Design review of the part built by this model. Coordinates are the model's own, in mm. A direction names the side the tool comes from. Give positions to 0.01 mm unless a question says otherwise; leave off trailing zeros. Write each loop counter-clockwise with the first axis right and the second up, starting at its lowest first coordinate (ties: lowest second). Pieces come first, ordered by that corner, then holes. Notation, with made-up numbers: M 30,65 L 84,65 A12 cw 84,72 Z; hole C 0.25,81.5 d6. An arc over 180 degrees is marked long. Write each question's results on one line, items separated by ' | '. Start each with the question number.
Autodesk Inventor part; units mm, degrees
ref_plane "YZ Plane" through (0, 0, 0) normal (1, 0, 0) x (0, 1, 0)
ref_plane "XZ Plane" through (0, 0, 0) normal (0, 1, 0) x (-1, 0, 0)
ref_plane "XY Plane" through (0, 0, 0) normal (0, 0, 1) x (1, 0, 0)
sketch "Sketch1" plane through (0, 0, 0) normal (0, 0, 1) x (1, 0, 0)
  line L0 (0, 0) -> (-6.8, 0)
  line L1 (-6.8, 0) -> (-6.8, 2.775)
  line L2 (-6.8, 2.775) -> (-5.2, 2.775)
  line L3 (-5.2, 2.775) -> (-5.2, 1.5)
  line L4 (-5.2, 1.5) -> (6.8, 1.5)
  line L5 (6.8, 1.5) -> (6.8, 0)
  line L6 (6.8, 0) -> (0, 0)
  dimension "d0" = 12
  dimension "d1" = 2.775
  dimension "d2" = 1.6
  dimension "d3" = 1.5
revolve "Revolution1" add sketch "Sketch1" angle 360 about axis through (0, 0, 0) along (-1, 0, 0)
sketch "Sketch2" plane through (-6.8, 0, 0) normal (-1, 0, 0) x (0, 0, 1)
  line L0 (-1.1547, 0) -> (-0.5774, 1)
  line L1 (-0.5774, 1) -> (0.5774, 1)
  line L2 (0.5774, 1) -> (1.1547, 0)
  line L3 (1.1547, 0) -> (0.5774, -1)
  line L4 (0.5774, -1) -> (-0.5774, -1)
  line L5 (-0.5774, -1) -> (-1.1547, 0)
  point P0 (0, 0)
  point P1 (0, 0)
  dimension "d5" = 2
extrude "Extrusion1" cut sketch "Sketch2" against normal blind 1.5
properties part number "M3x12"
Q1. The part is to be moulded in two halves that separate along Y. For faces 1 (the flat face through (-6.06, 0.51, 0.86)), 2 (the cylindrical face through (0.88, -1.5, 0.07)), 3 (the flat face through (6.8, 0, 0)), say which applies: pulls with the +Y half, pulls with the -Y half, needs draft (parallel to the pull), parting line crosses it, or undercut.
Q2. We need section D-D on z = 2.05. Write out the cut boundary in (x, y).
Q3. We need section C-C on x = 4.75. Write out the cut boundary in (y, z), and give its area (3 significant figures).
Q4. We need section B-B on y = 0.85. Write out the cut boundary in (x, z).
Q5. Wall thickness on line 1 along X through (y, z) = (2.45, 0.55); line 2 along X through (y, z) = (0.5, 0.65); line 3 along Z through (x, y) = (-5.75, -0.6): over which ranges is each line inside the solid? List them lowest first. Write a range as from..to.
Q6. We need section A-A on z = 0. Write out the cut boundary in (x, y) (3 decimals).
Q7. For pin 1 Ø0.6 at (y, z) = (0, 0.5) entering from -X; pin 2 Ø2 at (x, z) = (0, -1) entering from +Y; pin 3 Ø2 at (y, z) = (1, 1.5) entering from +X; pin 4 Ø2 at (x, y) = (5, -0.5) entering from +Z, all flat-tipped, find the tip position at first contact; note any pin that passes through.
Q8. For faces 4 (the flat face through (-6, 1, 0)), 5 (the cylindrical face through (-5.99, 1.49, 2.34)), 6 (the flat face through (-5.2, 1.2, 1.2)), list the 3-axis set-ups (+Z, -Z, +X, -X, +Y, -Y) from which the entire face can be reached by the end or side of a thin tool; tool diameter is ignored.
Answer sheet:
1) face 1: undercut | face 2: parting line crosses it | face 3: needs draft
2) outline: M -6.8,-1.87 L -5.2,-1.87 L -5.2,1.87 L -6.8,1.87 Z
3) outline: C 0,0 d3 | area: 7.07 mm^2
4) outline: M -6.8,-2.64 L -5.2,-2.64 L -5.2,-1.24 L 6.8,-1.24 L 6.8,1.24 L -5.2,1.24 L -5.2,2.64 L -6.8,2.64 L -6.8,0.66 L -5.3,0.66 L -5.3,-0.66 L -6.8,-0.66 Z
5) line 1: -6.8..-5.2 | line 2: -5.3..6.8 | line 3: -2.71..-0.81, 0.81..2.71
6) outline: M -6.8,-2.775 L -5.2,-2.775 L -5.2,-1.5 L 6.8,-1.5 L 6.8,1.5 L -5.2,1.5 L -5.2,2.775 L -6.8,2.775 L -6.8,1 L -5.3,1 L -5.3,-1 L -6.8,-1 Z
7) pin 1: x = -5.3 | pin 2: y = 1.5 | pin 3: x = 6.8 | pin 4: z = 1.5
8) face 4: -X | face 5: +X, -X | face 6: +X
